from build123d import *

# Parameters (mm, degrees)
BOSS_EXTRUDE1_DEPTH      = 5
BOSS_EXTRUDE1_DEPTH_BACK = 5


with BuildPart() as part:
    # Sketch3 → Boss-Extrude1 (new, two sides: drawn at the far end of the back side and taken through both)
    with BuildSketch(Plane.XY.offset(-BOSS_EXTRUDE1_DEPTH_BACK)):
        with BuildLine():
            Line((-148.773080728, 225.6468162), (-18.440943254, 55.845528153))
            ThreePointArc((-18.440943254, 55.845528153), (0, 46.75311932), (18.440943254, 55.845528153))
            Line((18.440943254, 55.845528153), (148.773080728, 225.6468162))
            ThreePointArc((148.773080728, 225.6468162), (168.290702347, 236.386792537), (189.171977646, 228.624255112))
            Line((189.171977646, 228.624255112), (228.624255112, 189.171977646))
            ThreePointArc((228.624255112, 189.171977646), (236.423365061, 168.873706393), (226.569637526, 149.489434791))
            Line((226.569637526, 149.489434791), (16.86048881, -20.767436459))
            ThreePointArc((16.86048881, -20.767436459), (0, -26.75), (-16.86048881, -20.767436459))
            Line((-16.86048881, -20.767436459), (-226.569637526, 149.489434791))
            ThreePointArc((-226.569637526, 149.489434791), (-236.423365061, 168.873706393), (-228.624255112, 189.171977646))
            Line((-228.624255112, 189.171977646), (-189.171977646, 228.624255112))
            ThreePointArc((-189.171977646, 228.624255112), (-168.30539851, 236.187390033), (-148.773080728, 225.6468162))
        make_face()
        with BuildLine():
            Line((-21.483790521, 54.062332516), (-151.815927996, 223.863620563))
            ThreePointArc((-151.815927996, 223.863620563), (-168.738130189, 232.90636594), (-186.69489822, 226.147175686))
            Line((-186.69489822, 226.147175686), (-226.147175686, 186.69489822))
            ThreePointArc((-226.147175686, 186.69489822), (-232.924931888, 169.054842525), (-224.361626158, 152.20909116))
            Line((-224.361626158, 152.20909116), (-14.652477443, -18.04778009))
            ThreePointArc((-14.652477443, -18.04778009), (0, -23.24688068), (14.652477443, -18.04778009))
            Line((14.652477443, -18.04778009), (224.361626158, 152.20909116))
            ThreePointArc((224.361626158, 152.20909116), (232.924931888, 169.054842525), (226.147175686, 186.69489822))
            Line((226.147175686, 186.69489822), (186.69489822, 226.147175686))
            ThreePointArc((186.69489822, 226.147175686), (168.738130189, 232.90636594), (151.815927996, 223.863620563))
            Line((151.815927996, 223.863620563), (21.483790521, 54.062332516))
            ThreePointArc((21.483790521, 54.062332516), (0, 43.25), (-21.483790521, 54.062332516))
        make_face(mode=Mode.SUBTRACT)
    extrude(amount=BOSS_EXTRUDE1_DEPTH + BOSS_EXTRUDE1_DEPTH_BACK)


solid = part.part
Geometry check sheet. Reference: the model listing, model coordinates, mm. A direction names the side the tool comes from. Give positions to 0.01 mm unless a question says otherwise; leave off trailing zeros. Order: outer loops, then holes, each group sorted by start corner. A loop starts at its lowest first (then second) coordinate and runs counter-clockwise, first axis right, second up.
1. Sectioned sample at D-D (y = 29). Record the boundary of the cut face in (x, z).
Completed:
outline: (-78.16, -5) - (-72.6, -5) - (-72.6, 5) - (-78.16, 5) - close; (72.6, -5) - (78.16, -5) - (78.16, 5) - (72.6, 5) - close
2. Sectioned sample at C-C (x = 199.5). Record the boundary of the cut face in (y, z).
Completed:
outline: (127.51, -5) - (132.02, -5) - (132.02, 5) - (127.51, 5) - close; (213.34, -5) - (218.3, -5) - (218.3, 5) - (213.34, 5) - close
3. Sectioned sample at A-A (z = 2.75). Record the boundary of the cut face in (x, y), then the cut area to 3 significant figures.
Completed:
outline: (-228.62, 189.17) arc R26.75 ccw to (-226.57, 149.49) - (-16.86, -20.77) arc R26.75 ccw to (16.86, -20.77) - (226.57, 149.49) arc R26.75 ccw to (228.62, 189.17) - (189.17, 228.62) arc R26.75 ccw to (148.77, 225.65) - (18.44, 55.85) arc R23.25 cw to (-18.44, 55.85) - (-148.77, 225.65) arc R27.14 ccw to (-189.17, 228.62) - close; hole (-226.15, 186.69) arc R23.25 ccw to (-224.36, 152.21) - (-14.65, -18.05) arc R23.25 ccw to (14.65, -18.05) - (224.36, 152.21) arc R23.25 ccw to (226.15, 186.69) - (186.69, 226.15) arc R23.25 ccw to (151.82, 223.86) - (21.48, 54.06) arc R26.75 cw to (-21.48, 54.06) - (-151.82, 223.86) arc R23.25 ccw to (-186.69, 226.15) - close
area: 4,650 mm2
4. Access from +Z, -Z, +X, -X, +Y, -Y to the whole of each face (thin tool, end or side, straight path). Record for faces 4 (the face through (-206.14, 206.7, -0.07)), 5 (the face through (-236.405, 168.561, -0.07)), 6 (the face through (-84.519, 141.935, -0.07)).
Completed:
face 4: +Z, -Z
face 5: +Z, -Z, -X
face 6: +Z, -Z, +Y
5. Draft check along X on faces 1 (the face through (236.438, 169.187, -0.07)), 2 (the face through (-0.222, -23.246, -0.07)), 3 (the face through (36, 76, 5)). Enter one of: pulls with the +X half, pulls with the -X half, needs draft (parallel to the pull), parting line crosses it, or undercut.
Completed:
face 1: pulls with the +X half
face 2: undercut
face 3: needs draft
6. Depth check by flat-ended pin: pin 1 (4 mm diameter, centred on y = 50, z = 3, fed in from -X); pin 2 (6 mm diameter, centred on x = -139.5, z = -1.5, fed in from -Y); pin 3 (2 mm diameter, centred on y = 33, z = 2.5, fed in from -X). Enter the tip coordinate at first touch or a pass-through.
Completed:
pin 1: stops at x = -106.49
pin 2: stops at y = 76.36
pin 3: stops at x = -84.32
7. Sectioned sample at B-B (y = 88.5). Record the boundary of the cut face in (x, z), then the cut area to 3 significant figures.
Completed:
outline: (-151.45, -5) - (-145.89, -5) - (-145.89, 5) - (-151.45, 5) - close; (-47.92, -5) - (-43.51, -5) - (-43.51, 5) - (-47.92, 5) - close; (43.51, -5) - (47.92, -5) - (47.92, 5) - (43.51, 5) - close; (145.89, -5) - (151.45, -5) - (151.45, 5) - (145.89, 5) - close
area: 199 mm2
8. Scan lines: line 1 (X direction, y = 74.5, z = -4); line 2 (X direction, y = 177.5, z = -0.25); line 3 (Y direction, x = 213.5, z = -3.75). Record each from-to range of solid material in increasing order.
Completed:
line 1: x = -134.2 to -128.65, -37.17 to -32.76, 32.76 to 37.17, 128.65 to 134.2
line 2: x = -235.46 to -231.8, -116.23 to -111.82, 111.82 to 116.23, 231.8 to 235.46
line 3: y = 138.88 to 143.39, 199.34 to 204.3
